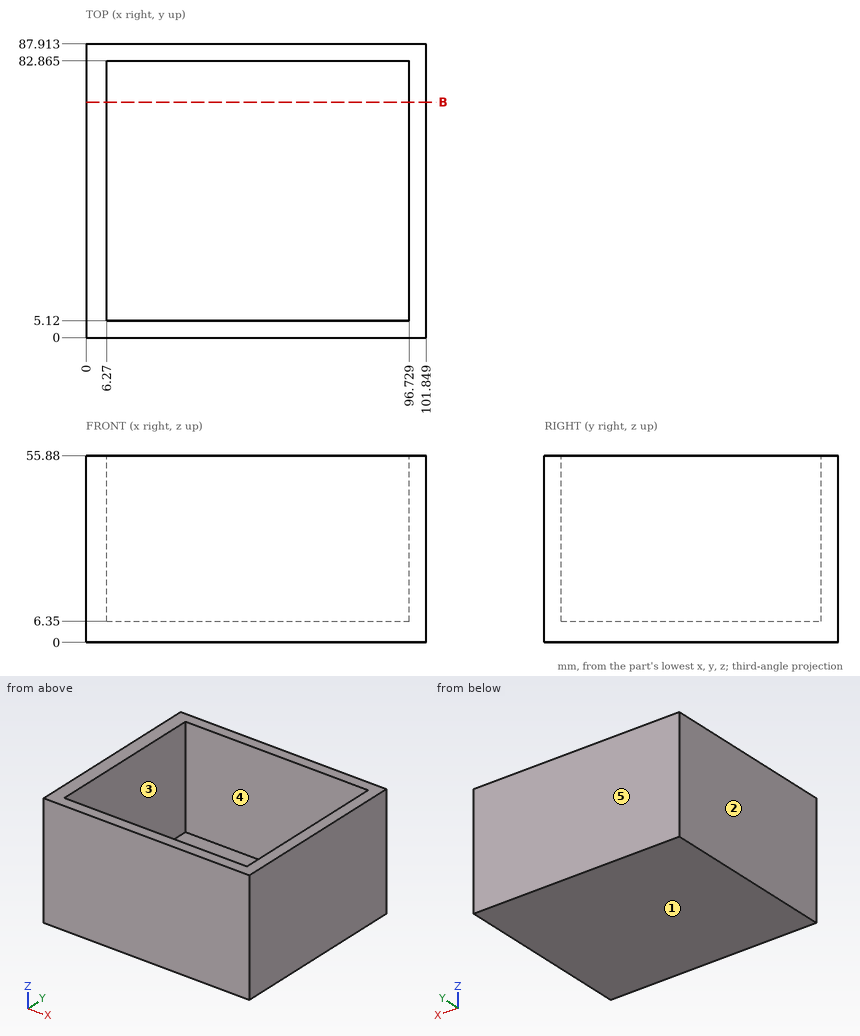
Drawing for the job (mm, zero at the part's lowest x, y, z). A direction names the side the tool comes from. Give positions to 0.01 mm unless a question says otherwise; leave off trailing zeros. Order: outer loops, then holes, each group sorted by start corner. A loop starts at its lowest first (then second) coordinate and runs counter-clockwise, first axis right, second up. Notation, with made-up numbers: M -23.5,23.5 L 33.5,23.5 A22 ccw 33.5,38.5 Z; hole C 67.5,-10.5 d5. An arc over 180 degrees is marked long. Put each result on its own line as item: value. Start each with the question number.
(1) Flat gauge pin, fed straight in: pin 1 Ø5 at (x, y) = (21.5, 59.5) entering from +Z. Where does the tip first touch, or does it go through?
(2) Which spindle directions (+Z, -Z, +X, -X, +Y, -Y) get a long thin tool onto all of the face, cutting with end or side? Do the marked faces 4 and 5. Say none if no direction does.
(3) Saw through at B-B, the plane y = 70.5. Write the cut outline in (x, z).
(4) Mould opens along X. For the marked faces 1, 2 and 3 say: +X half, -X half, draft (parallel to the pull), parting line (faces both ways), or undercut.
(5) Drill centre lines: line 1 along X through (y, z) = (37, 15.5); line 2 along Y through (x, z) = (62.5, 44) (1 decimal); line 3 along Z through (x, y) = (25, 63.5). Where is each one in solid material? Low to high.
Check result:
1. pin 1: stops at z = 6.35
2. face 4: +Z
2. face 5: +Z, -Z, +X, -X, +Y
3. outline: M 0,0 L 101.85,0 L 101.85,55.88 L 96.73,55.88 L 96.73,6.35 L 6.27,6.35 L 6.27,55.88 L 0,55.88 Z
4. face 1: draft
4. face 2: -X half
4. face 3: undercut
5. line 1: x = 0 to 6.27, 96.73 to 101.85
5. line 2: y = 0 to 5.1, 82.9 to 87.9
5. line 3: z = 0 to 6.35
